For this review, take the finished solid that the model builds, in its own axes (mm). Face numbers are marked on the shaded views. A direction names the side the tool comes from. Coordinates: 2 decimals unless noted, no trailing zeros. Write each loop counter-clockwise with the first axis right and the second up, starting at its lowest first coordinate (ties: lowest second). Pieces come first, ordered by that corner, then holes.
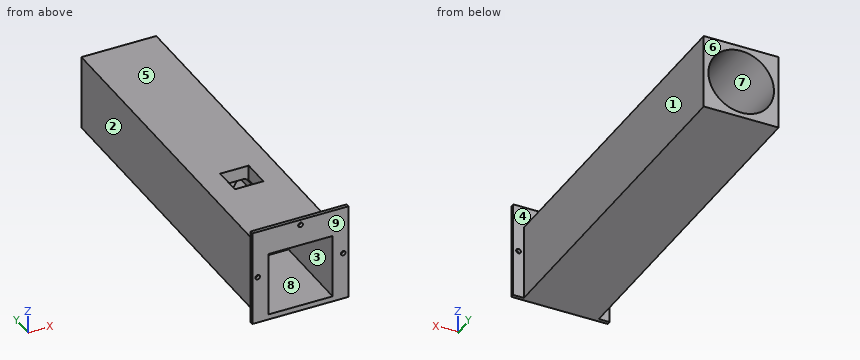
```python
from build123d import *

# Parameters (mm, degrees)
BOSS_EXTRUDE1_DEPTH = 50
BOSS_EXTRUDE2_START = 50
SKETCH2_3_R         = 23
BOSS_EXTRUDE2_DEPTH = 127.5
BOSS_EXTRUDE3_DEPTH = 177.5
SKETCH3_W           = 52.5
SKETCH3_H           = 52.5
BOSS_EXTRUDE4_DEPTH = 70
SKETCH6_W           = 20
SKETCH6_H           = 20
CUT_EXTRUDE7_DEPTH  = 30
SKETCH5_W           = 67.5
SKETCH5_H           = 67.5
SKETCH5_R           = 1.65
SKETCH5_W_2         = 47.5
SKETCH5_H_2         = 47.5
BOSS_EXTRUDE7_DEPTH = 2.5
SKETCH8_W           = 45
SKETCH8_H           = 45
CUT_EXTRUDE9_DEPTH  = 60


with BuildPart() as part:
    # Sketch2 → Boss-Extrude1 (new body)
    with BuildSketch(Plane(origin=(0, 0, 0), x_dir=(1, 0, 0), z_dir=(0, 1, 0))):
        with BuildLine():
            ThreePointArc((-26.25, -11.459990061), (-20.253319138, -20.253319138), (-11.459990061, -26.25))
            Line((-11.459990061, -26.25), (11.459990061, -26.25))
            ThreePointArc((11.459990061, -26.25), (20.253319138, -20.253319138), (26.25, -11.459990061))
            Line((26.25, -11.459990061), (26.25, 11.459990061))
            ThreePointArc((26.25, 11.459990061), (20.253319138, 20.253319138), (11.459990061, 26.25))
            Line((11.459990061, 26.25), (-11.459990061, 26.25))
            ThreePointArc((-11.459990061, 26.25), (-20.253319138, 20.253319138), (-26.25, 11.459990061))
            Line((-26.25, 11.459990061), (-26.25, -11.459990061))
        make_face()
        Polygon((-7.1, 17.237560734), (7.1, 17.237560734), (11.378165495, 14.767560734), (18.478165495, 2.47), (18.478165495, -2.47), (11.378165495, -14.767560734), (7.1, -17.237560734), (-7.1, -17.237560734), (-11.378165495, -14.767560734), (-18.478165495, -2.47), (-18.478165495, 2.47), (-11.378165495, 14.767560734), align=None, mode=Mode.SUBTRACT)
    extrude(amount=BOSS_EXTRUDE1_DEPTH)

    # Sketch2<3> → Boss-Extrude2 (add)
    with BuildSketch(Plane(origin=(0, 0, 0), x_dir=(1, 0, 0), z_dir=(0, 1, 0)).offset(BOSS_EXTRUDE2_START)):
        with BuildLine():
            ThreePointArc((-26.25, -11.459990061), (-20.253319138, -20.253319138), (-11.459990061, -26.25))
            Line((-11.459990061, -26.25), (11.459990061, -26.25))
            ThreePointArc((11.459990061, -26.25), (20.253319138, -20.253319138), (26.25, -11.459990061))
            Line((26.25, -11.459990061), (26.25, 11.459990061))
            ThreePointArc((26.25, 11.459990061), (20.253319138, 20.253319138), (11.459990061, 26.25))
            Line((11.459990061, 26.25), (-11.459990061, 26.25))
            ThreePointArc((-11.459990061, 26.25), (-20.253319138, 20.253319138), (-26.25, 11.459990061))
            Line((-26.25, 11.459990061), (-26.25, -11.459990061))
        make_face()
        with Locations(Location((0, 0, 0), (0, 0, 270))):
            Circle(SKETCH2_3_R, mode=Mode.SUBTRACT)
    extrude(amount=BOSS_EXTRUDE2_DEPTH)

    # Sketch2<4> → Boss-Extrude3 (add)
    with BuildSketch(Plane(origin=(0, 0, 0), x_dir=(1, 0, 0), z_dir=(0, 1, 0))):
        with BuildLine():
            Line((-26.25, 26.25), (-26.25, 11.459990061))
            ThreePointArc((-26.25, 11.459990061), (-20.253319138, 20.253319138), (-11.459990061, 26.25))
            Line((-11.459990061, 26.25), (-26.25, 26.25))
        make_face()
        with BuildLine():
            ThreePointArc((11.459990061, 26.25), (20.253319138, 20.253319138), (26.25, 11.459990061))
            Line((26.25, 11.459990061), (26.25, 26.25))
            Line((26.25, 26.25), (11.459990061, 26.25))
        make_face()
        with BuildLine():
            ThreePointArc((26.25, -11.459990061), (20.253319138, -20.253319138), (11.459990061, -26.25))
            Line((11.459990061, -26.25), (26.25, -26.25))
            Line((26.25, -26.25), (26.25, -11.459990061))
        make_face()
        with BuildLine():
            Line((-26.25, -11.459990061), (-26.25, -26.25))
            Line((-26.25, -26.25), (-11.459990061, -26.25))
            ThreePointArc((-11.459990061, -26.25), (-20.253319138, -20.253319138), (-26.25, -11.459990061))
        make_face()
    extrude(amount=BOSS_EXTRUDE3_DEPTH)

    # Sketch3 → Boss-Extrude4 (add)
    with BuildSketch(Plane.XZ):
        Rectangle(SKETCH3_W, SKETCH3_H)
    extrude(amount=BOSS_EXTRUDE4_DEPTH)

    # Sketch6 → Cut-Extrude7 (cut)
    with BuildSketch(Plane.XY.offset(26.25)):
        with Locations((0, 10)):
            Rectangle(SKETCH6_W, SKETCH6_H)
    extrude(amount=-CUT_EXTRUDE7_DEPTH, mode=Mode.SUBTRACT)

    # Sketch5 → Boss-Extrude7 (add)
    with BuildSketch(Plane.XZ.offset(70)):
        with Locations((0, 7.5)):
            Rectangle(SKETCH5_W, SKETCH5_H)
        with Locations(Location((0, 37.5, 0), (0, 0, 270))):
            Circle(SKETCH5_R, mode=Mode.SUBTRACT)
        with Locations(Location((-30, 7.5, 0), (0, 0, 270))):
            Circle(SKETCH5_R, mode=Mode.SUBTRACT)
        with Locations(Location((30, 7.5, 0), (0, 0, 270))):
            Circle(SKETCH5_R, mode=Mode.SUBTRACT)
        Rectangle(SKETCH5_W_2, SKETCH5_H_2, mode=Mode.SUBTRACT)
    extrude(amount=-BOSS_EXTRUDE7_DEPTH)

    # Sketch8 → Cut-Extrude9 (cut)
    with BuildSketch(Plane.XZ.offset(70)):
        Rectangle(SKETCH8_W, SKETCH8_H)
    extrude(amount=-CUT_EXTRUDE9_DEPTH, mode=Mode.SUBTRACT)


solid = part.part
```
Q1. Add section A-A (y = 134). State the section outline as (x, z) points, then the cut area to 3 significant figures.
Ans:
outline: (-26.25, -26.25) - (26.25, -26.25) - (26.25, 26.25) - (-26.25, 26.25) - close; hole circle Ø46 at (0, 0)
area: 1,090 mm2
Q2. Tool access review of the marked faces 5, 6, 7, 8 and 9: name each direction out of +Z, -Z, +X, -X, +Y, -Y from which nothing blocks a thin tool from reaching the whole face with its end or side.
Ans:
face 5: +Z, +X, -X, +Y
face 6: +Z, -Z, +X, -X, +Y
face 7: +Y
face 8: -Y
face 9: +Z, -Z, +X, -X, -Y
Q3. Draft analysis for pull direction X (two halves, no side actions). For the marked faces 1, 2, 3 and 4, state which applies: +X half, -X half, draft (parallel to the pull), parting line (faces both ways), or undercut.
Ans:
face 1: +X half
face 2: -X half
face 3: undercut
face 4: draft
Q4. Add section C-C (z = 31.5). State the section outline as (x, y) points.
Ans:
outline: (-33.75, -70) - (33.75, -70) - (33.75, -67.5) - (-33.75, -67.5) - close
Q5. Clearance check with flat-ended pins moving along their axes: pin 1 Ø3 at (x, z) = (19.5, 17) entering from -Y; pin 2 Ø2.5 at (y, z) = (37, -0.5) entering from +X; pin 3 Ø6 at (x, y) = (20.5, -17) entering from +Z; pin 4 Ø2.5 at (x, z) = (0, 37.5) entering from +Y. State where each tip first meets the part, or that it passes through.
Ans:
pin 1: stops at y = -10
pin 2: stops at x = 26.25
pin 3: stops at z = 26.25
pin 4: passes through
Q6. For probe 1 along Z at (x, y) = (5, 161); probe 2 along X at (y, z) = (119, 0); probe 3 along X at (y, z) = (-69.15, 37.5), list the stretches that pass through material, from the lowest coordinate up.
Ans:
probe 1: z = -26.25 to -22.45, 22.45 to 26.25
probe 2: x = -26.25 to -23, 23 to 26.25
probe 3: x = -33.75 to -1.65, 1.65 to 33.75
Q7. Add section B-B (z = 0). State the section outline as (x, y) points, then the cut area to 3 significant figures.
Ans:
outline: (-33.75, -70) - (-22.5, -70) - (-22.5, -10) - (22.5, -10) - (22.5, -70) - (33.75, -70) - (33.75, -67.5) - (26.25, -67.5) - (26.25, 177.5) - (23, 177.5) - (23, 50) - (18.48, 50) - (18.48, 0) - (-18.48, 0) - (-18.48, 50) - (-23, 50) - (-23, 177.5) - (-26.25, 177.5) - (-26.25, -67.5) - (-33.75, -67.5) - close
area: 2,620 mm2
